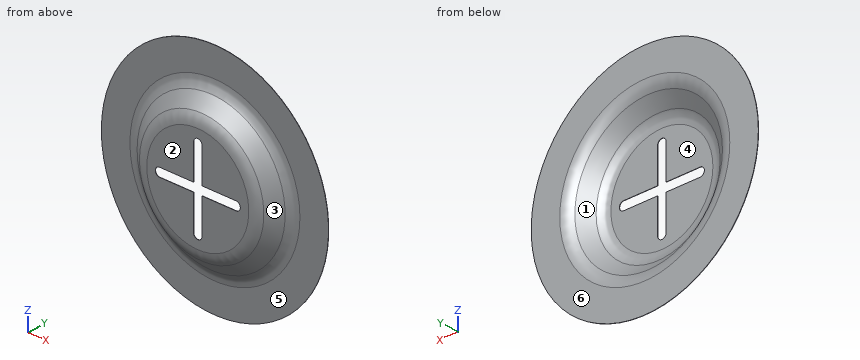
Autodesk Inventor part; units mm, degrees
ref_plane "YZ Plane" through (0, 0, 0) normal (1, 0, 0) x (0, 1, 0)
ref_plane "XZ Plane" through (0, 0, 0) normal (0, 1, 0) x (-1, 0, 0)
ref_plane "XY Plane" through (0, 0, 0) normal (0, 0, 1) x (1, 0, 0)
sketch "Skizze1" plane through (0, 0, 0) normal (0, 0, 1) x (1, 0, 0)
  line L0 (0, 0) -> (0, -0.02)
  line L1 (0, -0.02) -> (-3, -0.02)
  arc A0 (-3.6591, 0.2279) -> (-3, -0.02) centre (-3, 0.98) ccw
  line L2 (-3.6591, 0.2279) -> (-4.3541, 0.837)
  arc A1 (-4.3541, 0.837) -> (-5, 1.08) centre (-5, 0.1) ccw
  line L3 (-5, 1.08) -> (-6.68, 1.08)
  line L4 (-6.68, 1.08) -> (-6.68, 1.1)
  line L5 (-6.68, 1.1) -> (-5, 1.1)
  arc A2 (-4.3409, 0.8521) -> (-5, 1.1) centre (-5, 0.1) ccw
  line L6 (-4.3409, 0.8521) -> (-3.6459, 0.243)
  line L7 (-3, 0) -> (0, 0)
  arc A3 (-3.6459, 0.243) -> (-3, 0) centre (-3, 0.98) ccw
  dimension "d0" = 0.02
  dimension "d2" = 10
  dimension "d3" = 0.02
  dimension "d4" = 1
  dimension "d5" = 1.1
  dimension "d6" = 6
revolve "Umdrehung1" add sketch "Skizze1" angle 360 about axis through (0, 0, 0) along (0, -1, 0)
sketch "Skizze2" plane through (0, -0.02, 0) normal (0, -1, 0) x (1, 0, 0)
  line L0 (0, 0) -> (0, 2.5)
  line L1 (0, 2.5) -> (0.25, 2.5)
  line L2 (0.25, 2.5) -> (0.25, 0.25)
  line L3 (0.25, 0.25) -> (2.5, 0.25)
  line L4 (2.5, 0.25) -> (2.5, 0)
  line L5 (2.5, 0) -> (0, 0)
  arc A0 (2.5, 0) -> (2.25, 0.25) centre (2.25, 0) ccw
  arc A1 (0.25, 2.25) -> (0, 2.5) centre (0, 2.25) ccw
  arc A2 (-2.25, 0.25) -> (-2.5, 0) centre (-2.25, 0) ccw
  line L6 (-2.5, 0.25) -> (-0.25, 0.25)
  line L7 (-0.25, 2.5) -> (0, 2.5)
  arc A3 (0, 2.5) -> (-0.25, 2.25) centre (0, 2.25) ccw
  line L8 (-0.25, 0.25) -> (-0.25, 2.5)
  line L9 (-2.5, 0) -> (-2.5, 0.25)
  arc A4 (-0.25, -2.25) -> (0, -2.5) centre (0, -2.25) ccw
  line L10 (-0.25, -2.5) -> (-0.25, -0.25)
  line L11 (-2.5, -0.25) -> (-2.5, 0)
  arc A5 (-2.5, 0) -> (-2.25, -0.25) centre (-2.25, 0) ccw
  line L12 (-0.25, -0.25) -> (-2.5, -0.25)
  line L13 (0, -2.5) -> (-0.25, -2.5)
  arc A6 (2.25, -0.25) -> (2.5, 0) centre (2.25, 0) ccw
  line L14 (2.5, -0.25) -> (0.25, -0.25)
  line L15 (0.25, -2.5) -> (0, -2.5)
  arc A7 (0, -2.5) -> (0.25, -2.25) centre (0, -2.25) ccw
  line L16 (0.25, -0.25) -> (0.25, -2.5)
  line L17 (2.5, 0) -> (2.5, -0.25)
  point P0 (0, 2.5)
  point P1 (-2.5, 0)
  point P2 (0, -2.5)
  point P3 (2.5, 0)
  dimension "d8" = 5
  dimension "d9" = 0.5
  dimension "d12" = 360
extrude "Extrusion1" cut sketch "Skizze2" against normal through all contours L5 A6 L14 L16 A7 A4 L10 L12 A5 A2 L6 L8 A3 L0 | L0 A1 L2 L3 A0 L5
equation "\"d3\" = d0"
equation "\"Biegeradius\" = Stärke"
equation "\"BreiteBiegungsfreistellung\" = Stärke"
equation "\"TiefeBiegungsfreistellung\" = 0.5 * Stärke"
equation "\"GrößeEckenfreistellung\" = 4 * Stärke"
equation "\"MinimalRest\" = 2 * Stärke"
equation "\"Übergangsradius\" = Biegeradius"
equation "\"JacobiRadiusGröße\" = Biegeradius"
equation "\"Abstandsgröße\" = Stärke"
properties part number "bat_contacts_v2_contact_round"
Source: CAD feature listing. Evaluate the final solid. Frame: model axes, mm. Face numbers are marked on the shaded views. A direction names the side the tool comes from. Round coordinates to 2 decimals unless told otherwise and drop trailing zeros. Loops run counter-clockwise (first coordinate to the right, second up) from the corner with the lowest first, then second, coordinate; pieces in that order, holes last.
Q1. Section C-C, the plane y = 0.45. Return loops of the section in (x, z).
Q2. Access query for the marked faces 5 and 6. Directions: +Z, -Z, +X, -X, +Y, -Y. A direction counts if a zero-diameter tool reaches every point of the face in a straight line with its end or side. Return the directions, or none.
Q3. First-contact query: P1, Ø1.8, axis at x = -1, z = 0.5, coming from the +Y side; P2, Ø1.5, axis at x = 2.5, z = 2, coming from the +Y side; P3, Ø4, axis at x = 0.5, z = 2, coming from the +Y side. Flat tips, straight axial feed; report the tip coordinate or a pass-through.
Q4. Mould query, pull axis X, two halves, no side actions, for the marked faces 1, 2, 3 and 4. Classes: pulls with the +X half, pulls with the -X half, needs draft (parallel to the pull), parting line crosses it, or undercut.
Solutions:
1. outline: circle Ø7.83 at (0, 0); hole circle Ø7.76 at (0, 0)
2. face 5: -Y
2. face 6: +Z, -Z, +X, -X, +Y
3. P1: stops at y = 0
3. P2: stops at y = 0.51
3. P3: stops at y = 0.61
4. face 1: undercut
4. face 2: needs draft
4. face 3: parting line crosses it
4. face 4: undercut
